The listing builds one solid part. Answer for the finished solid, in the listing's coordinates (mm). A direction names the side the tool comes from. Give positions to 0.01 mm unless a question says otherwise; leave off trailing zeros. Order: outer loops, then holes, each group sorted by start corner. A loop starts at its lowest first (then second) coordinate and runs counter-clockwise, first axis right, second up. Notation, with made-up numbers: (-8.75, 5.25) - (46.25, 5.25) arc R8 ccw to (46.25, 17.25) - close; hole circle Ø5 at (62.25, 8). An arc over 180 degrees is marked (long way). Answer in a Markdown table with one row per item.
from build123d import *

# Parameters (mm, degrees)
ESQUISSE1_W             = 110
ESQUISSE1_H             = 100
BOSS_EXTRU_1_DEPTH      = 60
CONG_1_R                = 5
ESQUISSE2_W             = 102.640200382
ESQUISSE2_H             = 92.45985442
ENL_V_MAT_EXTRU_1_DEPTH = 55
CONG_2_R                = 5
ESQUISSE3_W             = 11.37967439
ESQUISSE3_H             = 5.215684095
ESQUISSE3_W_2           = 11.498212665
ESQUISSE3_W_3           = 11.261136116
ESQUISSE3_W_4           = 10.905521291
ENL_V_MAT_EXTRU_2_DEPTH = 55
CONG_3_R                = 1
ESQUISSE4_W             = 6.250199949
ESQUISSE4_H             = 8.836489583
ENL_V_MAT_EXTRU_3_DEPTH = 55
CONG_4_R                = 1
ESQUISSE6_W             = 129.088181363
ESQUISSE6_H             = 36.035635569
ENL_V_MAT_EXTRU_5_DEPTH = 115


with BuildPart() as part:
    # Esquisse1 → Boss.-Extru.1 (new body)
    with BuildSketch(Plane.XY):
        with Locations((-55, 50)):
            Rectangle(ESQUISSE1_W, ESQUISSE1_H)
    extrude(amount=BOSS_EXTRU_1_DEPTH)

    # Congé1
    cong_1_edges = [part.edges().sort_by_distance(p)[0] for p in [
        (0, 0, 30),
        (-110, 0, 30),
        (-110, 100, 30),
        (0, 100, 30),
    ]]
    fillet(cong_1_edges, radius=CONG_1_R)

    # Esquisse2 → Enlèv. mat.-Extru.1 (cut)
    with BuildSketch(Plane.XY.offset(60)):
        with Locations((-55, 50)):
            Rectangle(ESQUISSE2_W, ESQUISSE2_H)
    extrude(amount=-ENL_V_MAT_EXTRU_1_DEPTH, mode=Mode.SUBTRACT)

    # Congé2
    cong_2_edges = [part.edges().sort_by_distance(p)[0] for p in [
        (-106.320100191, 3.77007279, 32.5),
        (-106.320100191, 96.22992721, 32.5),
        (-3.679899809, 96.22992721, 32.5),
        (-3.679899809, 3.77007279, 32.5),
    ]]
    fillet(cong_2_edges, radius=CONG_2_R)

    # Esquisse3 → Enlèv. mat.-Extru.2 (cut)
    with BuildSketch(Plane.XZ):
        with Locations((-81.552573577, 12.752681003)):
            Rectangle(ESQUISSE3_W, ESQUISSE3_H)
        with Locations((-63.356948381, 12.752681003)):
            Rectangle(ESQUISSE3_W_2, ESQUISSE3_H)
        with Locations((-47.354281269, 12.752681003)):
            Rectangle(ESQUISSE3_W_3, ESQUISSE3_H)
        with Locations((-32.359189495, 12.752681003)):
            Rectangle(ESQUISSE3_W_4, ESQUISSE3_H)
    extrude(amount=-ENL_V_MAT_EXTRU_2_DEPTH, mode=Mode.SUBTRACT)

    # Congé3
    cong_3_edges = [part.edges().sort_by_distance(p)[0] for p in [
        (-69.106054713, 1.885036395, 10.144838955),
        (-69.106054713, 1.885036395, 15.36052305),
        (-57.607842048, 1.885036395, 15.36052305),
        (-57.607842048, 1.885036395, 10.144838955),
        (-52.984849327, 1.885036395, 10.144838955),
        (-52.984849327, 1.885036395, 15.36052305),
        (-41.723713211, 1.885036395, 15.36052305),
        (-41.723713211, 1.885036395, 10.144838955),
        (-37.81195014, 1.885036395, 10.144838955),
        (-37.81195014, 1.885036395, 15.36052305),
        (-26.906428849, 1.885036395, 15.36052305),
        (-26.906428849, 1.885036395, 10.144838955),
        (-87.242410772, 1.885036395, 10.144838955),
        (-87.242410772, 1.885036395, 15.36052305),
        (-75.862736382, 1.885036395, 15.36052305),
        (-75.862736382, 1.885036395, 10.144838955),
    ]]
    fillet(cong_3_edges, radius=CONG_3_R)

    # Esquisse4 → Enlèv. mat.-Extru.3 (cut)
    with BuildSketch(Plane.ZY.offset(110)):
        with Locations((13.781808753, 50.538810341)):
            Rectangle(ESQUISSE4_W, ESQUISSE4_H)
    extrude(amount=-ENL_V_MAT_EXTRU_3_DEPTH, mode=Mode.SUBTRACT)

    # Congé4
    cong_4_edges = [part.edges().sort_by_distance(p)[0] for p in [
        (-108.160050095, 46.120565549, 16.906908727),
        (-108.160050095, 46.120565549, 10.656708778),
        (-108.160050095, 54.957055132, 10.656708778),
        (-108.160050095, 54.957055132, 16.906908727),
    ]]
    fillet(cong_4_edges, radius=CONG_4_R)

    # Esquisse6 → Enlèv. mat.-Extru.5 (cut)
    with BuildSketch(Plane(origin=(0, 0, 0), x_dir=(1, 0, 0), z_dir=(0, 1, 0))):
        with Locations((-55.445822543, -49.658229713)):
            Rectangle(ESQUISSE6_W, ESQUISSE6_H)
    extrude(amount=ENL_V_MAT_EXTRU_5_DEPTH, mode=Mode.SUBTRACT)


solid = part.part
Item 1: Find section B-B on y = 17.5. Write down the section's boundary in (x, z).
Answer block:
| item | result |
|---|---|
| outline | (-110, 0) - (0, 0) - (0, 31.64) - (-3.68, 31.64) - (-3.68, 5) - (-106.32, 5) - (-106.32, 31.64) - (-110, 31.64) - close |
Item 2: Find section C-C on z = 7.5. Write down the section's boundary in (x, y), then the cut area to 3 significant figures.
Answer block:
| item | result |
|---|---|
| outline | (-110, 5) arc R5 ccw to (-105, 0) - (-5, 0) arc R5 ccw to (0, 5) - (0, 95) arc R5 ccw to (-5, 100) - (-105, 100) arc R5 ccw to (-110, 95) - close; hole (-106.32, 8.77) arc R5 ccw to (-101.32, 3.77) - (-8.68, 3.77) arc R5 ccw to (-3.68, 8.77) - (-3.68, 91.23) arc R5 ccw to (-8.68, 96.23) - (-101.32, 96.23) arc R5 ccw to (-106.32, 91.23) - close |
| area | 1,510 mm² |
Item 3: Determine the mould class of faces 1 (the face through (-106.32, 49, 19)), 2 (the face through (-108, 46.121, 14)), 3 (the face through (-109, 98, 16)), 4 (the face through (-63, 2, 15.361)) for opening direction Y: pulls with the +Y half, pulls with the -Y half, needs draft (parallel to the pull), parting line crosses it, or undercut.
Answer block:
| item | result |
|---|---|
| face 1 | undercut |
| face 2 | undercut |
| face 3 | pulls with the +Y half |
| face 4 | needs draft |
Item 4: Find section D-D on x = -93.5. Write down the section's boundary in (y, z), then the cut area to 3 significant figures.
Answer block:
| item | result |
|---|---|
| outline | (0, 0) - (100, 0) - (100, 31.64) - (96.23, 31.64) - (96.23, 5) - (3.77, 5) - (3.77, 31.64) - (0, 31.64) - close |
| area | 701 mm² |
Item 5: Consider line 1 (Y direction, x = -80, z = 7); line 2 (X direction, y = 82.5, z = 6); line 3 (Z direction, x = -99.5, y = 85). Determine where each line is inside the solid, lowest interval first.
Answer block:
| item | result |
|---|---|
| line 1 | 0 to 3.77, 96.23 to 100 |
| line 2 | -110 to -106.32, -3.68 to 0 |
| line 3 | 0 to 5 |
Item 6: Find section A-A on x = -49.5. Write down the section's boundary in (y, z).
Answer block:
| item | result |
|---|---|
| outline | (0, 0) - (100, 0) - (100, 31.64) - (96.23, 31.64) - (96.23, 5) - (3.77, 5) - (3.77, 10.14) - (0, 10.14) - close; (0, 15.36) - (3.77, 15.36) - (3.77, 31.64) - (0, 31.64) - close |
Item 7: Which of the six approach directions +Z, -Z, +X, -X, +Y, -Y give full straight-line access (tool end or side, diameter ignored) to faces 5 (the face through (-59, 98, 31.64)), 6 (the face through (-57.608, 2, 13)), 7 (the face through (0, 49, 16)), 8 (the face through (-108, 50, 10.657)), 9 (the face through (-104.82, 5.2, 18.13))?
Answer block:
| item | result |
|---|---|
| face 5 | +Z, +X, -X, +Y, -Y |
| face 6 | -Y |
| face 7 | +Z, -Z, +X, +Y, -Y |
| face 8 | -X |
| face 9 | +Z |
Item 8: Each of these flat-tipped pins is pushed along its axis until it touches: P1, Ø1, axis at y = 1, z = 12.5, coming from the -X side; P2, Ø5, axis at x = -73.5, y = 67.5, coming from the +Z side; P3, Ø2.5, axis at y = 2, z = 13.5, coming from the -X side. Where does it stop, or does it pass through?
Answer block:
| item | result |
|---|---|
| P1 | x = -108.57 |
| P2 | z = 5 |
| P3 | x = -109.68 |
